Input: part model. Units: mm. Frame: model coordinates. A direction names the side the tool comes from. Round coordinates to 2 decimals unless told otherwise and drop trailing zeros. Loops run counter-clockwise (first coordinate to the right, second up) from the corner with the lowest first, then second, coordinate; pieces in that order, holes last. Notation, with made-up numbers: M 39,44.25 L 90,44.25 A18 ccw 90,73.25 Z; hole C 80,-37.5 d9. An arc over 180 degrees is marked long. Return JSON: item names as keys, results as strings. Group by question number.
1) Mould query, pull axis X, two halves, no side actions, for faces 3 (the face through (12.8, 7, 3)), 4 (the face through (-12.8, 0, 7)), 5 (the face through (-7, 0.8, 6)), 6 (the face through (12.8, 0, 7)). Classes: +X half, -X half, draft (parallel to the pull), parting line (faces both ways), or undercut.
2) Contact query for flat-ended pins moving along their axis: P1, Ø6, axis at x = 9.5, y = -8.5, coming from the +Z side; P2, Ø3.5, axis at x = 5.5, z = 8, coming from the -Y side; P3, Ø0.8, axis at y = 0.5, z = 7, coming from the +X side. Output: stop coordinate, or through.
3) Material intervals for line 1 (Y direction, x = 9.5, z = 1.5); line 2 (X direction, y = 5, z = 4.5); line 3 (Z direction, x = 12.25, y = 4.5), sorted ascending. Write a range as from..to.
4) Section A-A (z = 11.25). Output: boundary loops of the cut face in (x, y).
5) Section B-B (y = -11.25). Output: boundary loops of the cut face in (x, z), plus the area to 4 significant figures.
6) Section C-C (z = 1.75). Output: boundary loops of the cut face in (x, y), plus the area to 3 significant figures.
7) Access query for faces 1 (the face through (0, 0, 11.9)), 2 (the face through (7, -6, 0.5)). Directions: +Z, -Z, +X, -X, +Y, -Y. A direction counts if a zero-diameter tool reaches every point of the face in a straight line with its end or side. Return the directions, or none.
from build123d import *

# Parameters (mm, degrees)
F1_DEPTH = 11.9
F0_W     = 27.6
F0_H     = 27.6
F2_DEPTH = 5
F3_W     = 27
F3_H     = 27
F4_DEPTH = 0.5
F5_SIZE  = 2


with BuildPart() as f1:
    # F0 (on Top) → F1 (new body)
    with BuildSketch(Plane.XY):
        Polygon((0.5, 13.1), (-0.5, 13.1), (-0.5, 0.8), (-12.8, 0.8), (-12.8, -0.2), (-0.5, -0.2), (-0.5, -12.5), (0.5, -12.5), (0.5, -0.2), (12.8, -0.2), (12.8, 0.8), (0.5, 0.8), align=None)
    extrude(amount=F1_DEPTH)

    # F0 (on Top) → F2 (join)
    with BuildSketch(Plane.XY):
        with Locations((0, 0.3)):
            Rectangle(F0_W, F0_H)
        Polygon((-12.8, 0.8), (-12.8, 13.1), (-0.5, 13.1), (0.5, 13.1), (12.8, 13.1), (12.8, 0.8), (12.8, -0.2), (12.8, -12.5), (0.5, -12.5), (-0.5, -12.5), (-12.8, -12.5), (-12.8, -0.2), align=None, mode=Mode.SUBTRACT)
    extrude(amount=F2_DEPTH)

    # F3 (on Top) → F4 (join)
    with BuildSketch(Plane.XY):
        Rectangle(F3_W, F3_H)
    extrude(amount=F4_DEPTH)

    # F5
    f5_edges = [f1.edges().sort_by_distance(p)[0] for p in [
        (0, 13.1, 11.9),
        (-12.8, 0.3, 11.9),
        (0, -12.5, 11.9),
        (12.8, 0.3, 11.9),
    ]]
    chamfer(f5_edges, length=F5_SIZE)


solid = f1.part
Returned:
{
 "1": {"face 3": "undercut", "face 4": "-X half", "face 5": "undercut", "face 6": "+X half"},
 "2": {"P1": "stops at z = 0.5", "P2": "stops at y = -0.2", "P3": "stops at x = 12.8"},
 "3": {"line 1": "y = -13.5..-12.5, -0.2..0.8, 13.1..14.1", "line 2": "x = -13.8..-12.8, -0.5..0.5, 12.8..13.8", "line 3": "z = 0..0.5"},
 "4": {"outline": "M -11.45,-0.2 L -0.5,-0.2 L -0.5,-11.15 L 0.5,-11.15 L 0.5,-0.2 L 11.45,-0.2 L 11.45,0.8 L 0.5,0.8 L 0.5,11.75 L -0.5,11.75 L -0.5,0.8 L -11.45,0.8 Z"},
 "5": {"outline": "M -13.8,0 L 13.8,0 L 13.8,5 L 12.8,5 L 12.8,0.5 L 0.5,0.5 L 0.5,11.15 L -0.5,11.15 L -0.5,0.5 L -12.8,0.5 L -12.8,5 L -13.8,5 Z", "area": "33.45 mm^2"},
 "6": {"outline": "M -13.8,-13.5 L 13.8,-13.5 L 13.8,14.1 L -13.8,14.1 Z; hole M -12.8,-12.5 L -0.5,-12.5 L -0.5,-0.2 L -12.8,-0.2 Z; hole M -12.8,0.8 L -0.5,0.8 L -0.5,13.1 L -12.8,13.1 Z; hole M 0.5,-12.5 L 12.8,-12.5 L 12.8,-0.2 L 0.5,-0.2 Z; hole M 0.5,0.8 L 12.8,0.8 L 12.8,13.1 L 0.5,13.1 Z", "area": "157 mm^2"},
 "7": {"face 1": "+Z, +X, -X, +Y, -Y", "face 2": "+Z"}
}
